```python
from build123d import *

# Parameters (mm, degrees)
SKETCH1_W           = 431.8
SKETCH1_H           = 285.75
BOSS_EXTRUDE1_DEPTH = 6.35
SKETCH2_W           = 431.8
SKETCH2_H           = 6.35
BOSS_EXTRUDE2_DEPTH = 12.7
CUT_EXTRUDE1_DEPTH  = 20.05
SKETCH5_W           = 33.462355894
SKETCH5_H           = 294.779483051
CUT_EXTRUDE2_DEPTH  = 432.8
SKETCH4_W           = 12.7
SKETCH4_H           = 6.35
CUT_EXTRUDE3_DEPTH  = 6.35


with BuildPart() as part:
    # Sketch1 → Boss-Extrude1 (new body)
    with BuildSketch(Plane(origin=(0, 0, 0), x_dir=(0, 0, -1), z_dir=(1, 0, 0))):
        Rectangle(SKETCH1_W, SKETCH1_H)
    extrude(amount=BOSS_EXTRUDE1_DEPTH)

    # Sketch2 → Boss-Extrude2 (add)
    with BuildSketch(Plane(origin=(6.35, 0, 0), x_dir=(0, 0, -1), z_dir=(1, 0, 0))):
        with Locations((0, 139.7)):
            Rectangle(SKETCH2_W, SKETCH2_H)
    extrude(amount=BOSS_EXTRUDE2_DEPTH)

    # Sketch3 → Cut-Extrude1 (cut, through all)
    with BuildSketch(Plane.ZY):
        with BuildLine():
            Line((-190.5, -85.725), (0, -85.725))
            ThreePointArc((0, -85.725), (12.7, -98.425), (0, -111.125))
            Line((0, -111.125), (-190.5, -111.125))
            ThreePointArc((-190.5, -111.125), (-203.2, -98.425), (-190.5, -85.725))
        make_face()
    extrude(amount=-CUT_EXTRUDE1_DEPTH, mode=Mode.SUBTRACT)

    # Sketch5 → Cut-Extrude2 (cut, through all)
    with BuildSketch(Plane(origin=(0, 0, -215.9), x_dir=(-1, 0, 0), z_dir=(0, 0, -1))):
        with Locations((10.381177947, -10.864741526)):
            Rectangle(SKETCH5_W, SKETCH5_H)
    extrude(amount=-CUT_EXTRUDE2_DEPTH, mode=Mode.SUBTRACT)

    # Sketch4 → Cut-Extrude3 (cut)
    with BuildSketch(Plane.ZY):
        with Locations((-183.35625, 139.7)):
            Rectangle(SKETCH4_W, SKETCH4_H)
        with Locations((-209.55, 139.7)):
            Rectangle(SKETCH4_W, SKETCH4_H)
        with Locations((-157.1625, 139.7)):
            Rectangle(SKETCH4_W, SKETCH4_H)
        with Locations((-130.96875, 139.7)):
            Rectangle(SKETCH4_W, SKETCH4_H)
        with Locations((-104.775, 139.7)):
            Rectangle(SKETCH4_W, SKETCH4_H)
        with Locations((-78.58125, 139.7)):
            Rectangle(SKETCH4_W, SKETCH4_H)
        with Locations((-52.3875, 139.7)):
            Rectangle(SKETCH4_W, SKETCH4_H)
        with Locations((-26.19375, 139.7)):
            Rectangle(SKETCH4_W, SKETCH4_H)
        with Locations((0, 139.7)):
            Rectangle(SKETCH4_W, SKETCH4_H)
        with Locations((26.19375, 139.7)):
            Rectangle(SKETCH4_W, SKETCH4_H)
        with Locations((52.3875, 139.7)):
            Rectangle(SKETCH4_W, SKETCH4_H)
        with Locations((78.58125, 139.7)):
            Rectangle(SKETCH4_W, SKETCH4_H)
        with Locations((104.775, 139.7)):
            Rectangle(SKETCH4_W, SKETCH4_H)
        with Locations((130.96875, 139.7)):
            Rectangle(SKETCH4_W, SKETCH4_H)
        with Locations((157.1625, 139.7)):
            Rectangle(SKETCH4_W, SKETCH4_H)
        with Locations((183.35625, 139.7)):
            Rectangle(SKETCH4_W, SKETCH4_H)
        with Locations((209.55, 139.7)):
            Rectangle(SKETCH4_W, SKETCH4_H)
    extrude(amount=-CUT_EXTRUDE3_DEPTH, mode=Mode.SUBTRACT)


solid = part.part
```
Design review of the part built by this model. Coordinates are the model's own, in mm. Give positions to 0.01 mm unless a question says otherwise; leave off trailing zeros. Write each loop counter-clockwise with the first axis right and the second up, starting at its lowest first coordinate (ties: lowest second). Pieces come first, ordered by that corner, then holes. Notation, with made-up numbers: (6, 0) - (60, 0) arc R15 cw to (60, 13) - close; hole circle Ø2 at (-24, 82.25). An arc over 180 degrees is marked (long way). Return JSON: item names as keys, results as strings. Group by question number.
(1) To check wall thickness, follow probe 1 along X at (y, z) = (139.75, 125.5). State the ranges of the line that lie inside material, in increasing order.
(2) Insertion check: pin 1 (1.9 mm diameter, centred on x = 4.5, y = 139, fed in from -Z); pin 2 (1.9 mm diameter, centred on x = 4, y = 139, fed in from +Z). Each pin has a flat end and moves straight along its axis. Give the tip position at first contact, or say it passes through.
(3) We need section B-B, the plane x = 3. Give the number of separate pieces and of enclosed holes in the cut face, then the cut area to 3 significant figures.
(4) We need section A-A, the plane z = -78. Give the boundary of the cut face in (x, y) (3 decimals), then the cut area to 3 significant figures.
Reported:
{
 "1": {"probe 1": "x = 6.35 to 19.05"},
 "2": {"pin 1": "stops at z = -203.2", "pin 2": "stops at z = 203.2"},
 "3": {"separate pieces": "16", "enclosed holes": "0", "area": "1,370 mm2"},
 "4": {"outline": "(6.35, 136.525) - (19.05, 136.525) - (19.05, 142.875) - (6.35, 142.875) - close", "area": "80.6 mm2"}
}
